Here's the drawing with two shaded views (mm, measured from the low corner). I have some questions. A direction names the side the tool comes from. Coordinates: 2 decimals unless noted, no trailing zeros. Write each loop counter-clockwise with the first axis right and the second up, starting at its lowest first coordinate (ties: lowest second). Pieces come first, ordered by that corner, then holes.
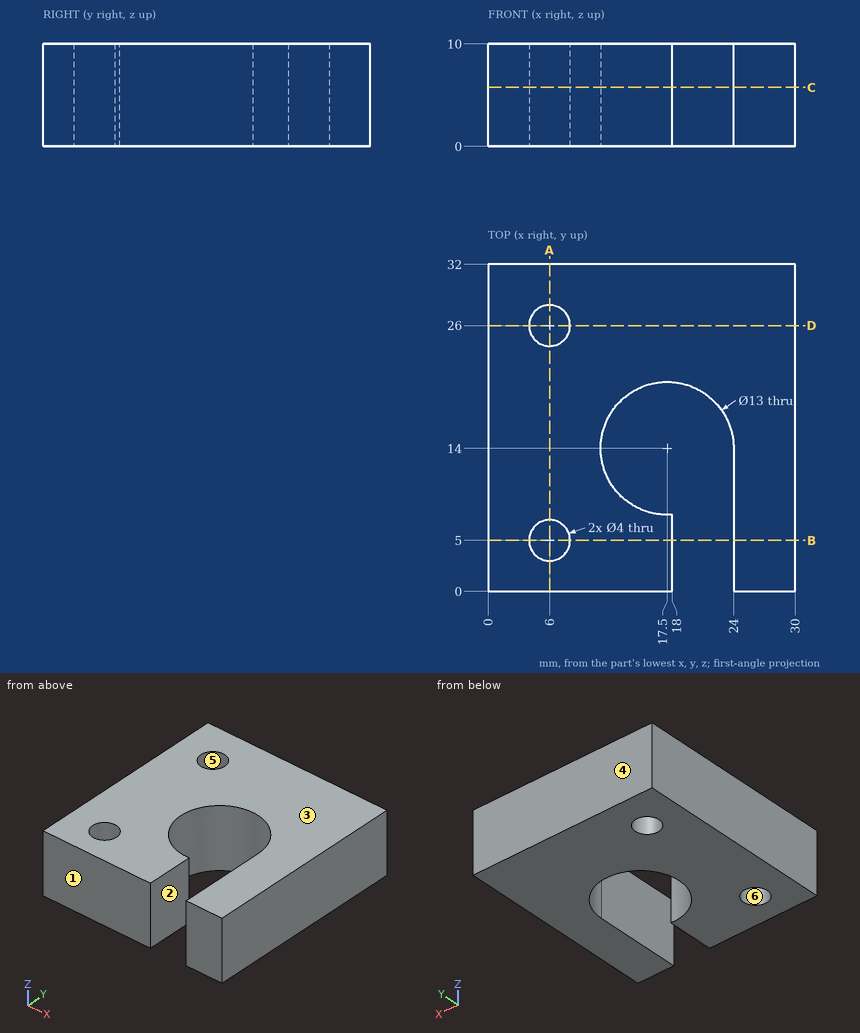
1. For pin 1 (5 mm diameter, centred on x = 6, y = 26, fed in from +Z); pin 2 (3 mm diameter, centred on x = 6, y = 5, fed in from -Z), each with a flat end and sliding along its axis, tell me the tip position at first contact or that it passes through.
Verdict:
pin 1: stops at z = 10
pin 2: passes through
2. If we mould it in two halves opening along Y, with no side actions, what happens to the marked faces 3, 4, 5 and 6? For each: pulls with the +Y half, pulls with the -Y half, needs draft (parallel to the pull), parting line crosses it, or undercut.
Verdict:
face 3: needs draft
face 4: pulls with the +Y half
face 5: undercut
face 6: undercut
3. I want a section at A-A on x = 6. Please give me the cut outline in (y, z), plus the area to 3 significant figures.
Verdict:
outline: (0, 0) - (3, 0) - (3, 10) - (0, 10) - close; (7, 0) - (24, 0) - (24, 10) - (7, 10) - close; (28, 0) - (32, 0) - (32, 10) - (28, 10) - close
area: 240 mm2
4. I want a section at D-D on y = 26. Please give me the cut outline in (x, z).
Verdict:
outline: (0, 0) - (4, 0) - (4, 10) - (0, 10) - close; (8, 0) - (30, 0) - (30, 10) - (8, 10) - close
5. I want a section at C-C on z = 5.75. Please give me the cut outline in (x, y), plus the area to 3 significant figures.
Verdict:
outline: (0, 0) - (18, 0) - (18, 7.52) arc R6.5 cw (long way) to (24, 14) - (24, 0) - (30, 0) - (30, 32) - (0, 32) - close; hole circle Ø4 at (6, 5); hole circle Ø4 at (6, 26)
area: 748 mm2
6. On a 3-axis mill with a long thin cutter (end or side, diameter ignored), from which of +Z, -Z, +X, -X, +Y, -Y can I reach the whole of each face in a straight line? I mean the marked faces 1 and 2. Say none if no direction works.
Verdict:
face 1: +Z, -Z, +X, -X, -Y
face 2: +Z, -Z, -Y
7. Please list where these lines run through material, in increasing order: line 1 along Y through (x, z) = (6, 6.5); line 2 along X through (y, z) = (14, 2.5); line 3 along Y through (x, z) = (17.5, 6.25).
Verdict:
line 1: y = 0 to 3, 7 to 24, 28 to 32
line 2: x = 0 to 11, 24 to 30
line 3: y = 0 to 7.5, 20.5 to 32
8. I want a section at B-B on y = 5. Please give me the cut outline in (x, z), plus the area to 3 significant figures.
Verdict:
outline: (0, 0) - (4, 0) - (4, 10) - (0, 10) - close; (8, 0) - (18, 0) - (18, 10) - (8, 10) - close; (24, 0) - (30, 0) - (30, 10) - (24, 10) - close
area: 200 mm2
